Geometry check sheet. Reference: the model listing, model coordinates, mm. Give positions to 0.01 mm unless a question says otherwise; leave off trailing zeros. Order: outer loops, then holes, each group sorted by start corner. A loop starts at its lowest first (then second) coordinate and runs counter-clockwise, first axis right, second up. Notation, with made-up numbers: M 51,68.25 L 110,68.25 A25 cw 110,101.25 Z; hole C 43,77.25 d3. An arc over 180 degrees is marked long. Answer as CSV lines item,"result". Start each with the question number.
Q1. Thickness scan on line 1 (Z direction, x = -110, y = 0.5); line 2 (X direction, y = 1.5, z = 110). Record the ranges inside material, lowest first.
Q2. Section check B-B, the plane x = -110. Record the boundary of the cut face in (y, z).
Q3. Go/stop test with a flat-tipped pin: pin 1 (7.5 mm diameter, centred on x = -110, z = 110, fed in from -Y). Record where the tip stops, or that it passes through.
Q4. Section check A-A, the plane z = 110. Record the boundary of the cut face in (x, y), then the cut area to 3 significant figures.
Autodesk Inventor part; units mm, degrees
ref_plane "YZ Plane" through (0, 0, 0) normal (1, 0, 0) x (0, 1, 0)
ref_plane "XZ Plane" through (0, 0, 0) normal (0, 1, 0) x (-1, 0, 0)
ref_plane "XY Plane" through (0, 0, 0) normal (0, 0, 1) x (1, 0, 0)
sketch "스케치1" plane through (0, 0, 0) normal (0, 1, 0) x (-1, 0, 0)
  line L0 (125, -125) -> (-125, -125)
  line L1 (-125, -125) -> (-125, 125)
  line L2 (-125, 125) -> (125, 125)
  line L3 (125, 125) -> (125, -125)
  point P0 (0, 0)
  point P1 (125, 0)
  point P2 (0, -125)
  dimension "d0" = 250
  dimension "d1" = 250
extrude "돌출1" add sketch "스케치1" along normal mid plane 12
sketch "Sketch2" plane through (0, 6, 0) normal (0, 1, 0) x (1, 0, 0)
  line L0 (-125, -125) -> (-95, -125)
  line L1 (-95, -125) -> (-95, -95)
  line L2 (-95, -95) -> (-125, -95)
  line L3 (-125, -95) -> (-125, -125)
  line L4 (-125, -95) -> (-95, -125)
  line L5 (-95, -95) -> (-125, -125)
  point P0 (0, 0)
  point P1 (-110, -110)
  point P2 (-95, -110)
  point P3 (-110, -95)
  dimension "d5" = 30
  dimension "d6" = 30
sketch "Sketch3" plane through (0, 6, 0) normal (0, 1, 0) x (1, 0, 0)
  line L0 (-125, -125) -> (-125, 125)
  line L1 (-125, 125) -> (-185, 125)
  line L2 (-185, 125) -> (-185, -125)
  line L3 (-185, -125) -> (-125, -125)
  line L4 (-125, -125) -> (-125, 125)
  point P0 (0, 0)
  dimension "d7" = 60
  dimension "d8" = 250
extrude "Extrusion2" add sketch "Sketch3" against normal up to surface (12 mm away)
sketch "Sketch4" plane through (0, -6, 0) normal (0, -1, 0) x (1, 0, 0)
  circle A0 centre (-110, 110) radius 2.5
  point P0 (0, 0)
hole "Hole1" at (-110, -6, 110) direction (0, 1, 0) diameter 6.6 end through all countersink diameter 12.6 countersink angle 90
equation "\"d1\" = d0"
equation "\"TransitionRadius\" = BendRadius"
properties part number "Base_Wood_Plate" material "Wood (Birch)"
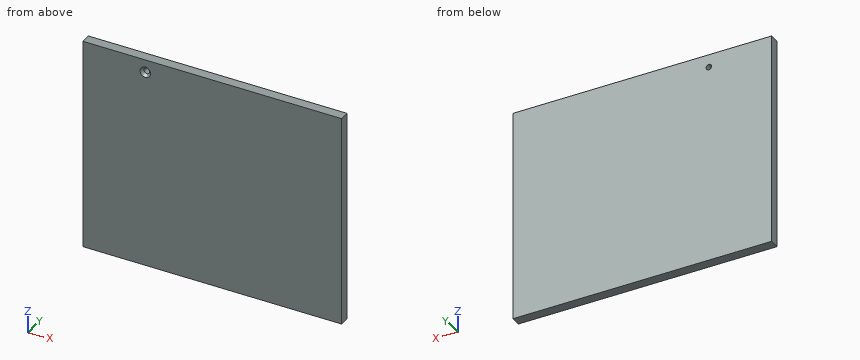
Answer block:
1,line 1,"z = -125 to 106.7, 113.3 to 125"
1,line 2,"x = -185 to -113.3, -106.7 to 125"
2,outline,"M -6,-125 L 6,-125 L 6,106.7 L -3,106.7 L -6,103.7 Z; M -6,116.3 L -3,113.3 L 6,113.3 L 6,125 L -6,125 Z"
3,pin 1,"stops at y = -3.45"
4,outline,"M -185,-6 L -116.3,-6 L -113.3,-3 L -113.3,6 L -185,6 Z; M -106.7,-3 L -103.7,-6 L 125,-6 L 125,6 L -106.7,6 Z"
4,area,"3,630 mm2"
